Design review of the part built by this model. Coordinates are the model's own, in mm. A direction names the side the tool comes from. Coordinates: 2 decimals unless noted, no trailing zeros. Order: outer loops, then holes, each group sorted by start corner. A loop starts at its lowest first (then second) coordinate and runs counter-clockwise, first axis right, second up. Notation, with made-up numbers: M -32.5,54.25 L 17.5,54.25 A36 ccw 17.5,91.25 Z; hole C -14,67.25 d10. An arc over 180 degrees is marked long. Answer in a Markdown table with one row per item.
from build123d import *

# Parameters (mm, degrees)
PAD_DEPTH           = 50
PAD001_DEPTH        = 50
CHAMFER_SIZE        = 5
SKETCH002_R         = 6
POCKET_DEPTH        = 30
SKETCH015_R         = 6
POCKET005_DEPTH     = 292.6279206635
LINEARPATTERN_COUNT = 4
LINEARPATTERN_PITCH = 166.6666666667


with BuildPart() as part:
    # Sketch → Pad (new body)
    with BuildSketch(Plane.XY):
        with BuildLine():
            Line((-447.460817474, 354.8217734667), (19.5015988359, 27.8511695058))
            ThreePointArc((34, 0), (30.1583683281, 15.69945285), (19.5015988359, 27.8511695058))
            Line((28, 0), (34, 0))
            ThreePointArc((28, 0), (24.836303329, 12.9289611706), (16.0601402178, 22.9362572401))
            Line((16.0601402178, 22.9362572401), (-450.9022760922, 349.906861201))
            Line((-450.9022760922, 349.906861201), (-447.460817474, 354.8217734667))
        make_face()
    extrude(amount=PAD_DEPTH)

    # Sketch001 → Pad001 (join)
    with BuildSketch(Plane.XY):
        Polygon((-94.6057566753, 107.75), (-103.1746447158, 113.75), (-1.7405688034, 113.75), (-1.7405688034, 107.75), align=None)
        Polygon((-113.171680763, 120.75), (-121.7405688034, 126.75), (-1.7405688034, 126.75), (-1.7405688034, 120.75), align=None)
    extrude(amount=PAD001_DEPTH)

    # Chamfer
    chamfer_edges = [part.edges().sort_by_distance(p)[0] for p in [
        (-1.740569, 123.75, 50),
        (-1.740569, 110.75, 50),
        (-1.740569, 110.75, 0),
        (-1.740569, 123.75, 0),
    ]]
    chamfer(chamfer_edges, length=CHAMFER_SIZE)

    # Sketch002 (on Face1 of Chamfer) → Pocket (cut)
    with BuildSketch(Plane(origin=(0, 126.75, 0), x_dir=(-1, 0, 0), z_dir=(0, 1, 0))):
        with Locations((26.7405688034, 25.24131)):
            Circle(SKETCH002_R)
    extrude(amount=-POCKET_DEPTH, mode=Mode.SUBTRACT)

    # Sketch015 → Pocket005 (cut, through all)
    with BuildSketch(Plane(origin=(19.5015988359, 27.8511695058, 0), x_dir=(-0.8191520443, 0.5735764364, 0), z_dir=(0.5735764364, 0.8191520443, 0))):
        with Locations((550.0558517379, 25)):
            Circle(SKETCH015_R)
    pocket005 = extrude(amount=-POCKET005_DEPTH, mode=Mode.SUBTRACT)

    # LinearPattern: Pocket005 ×4
    with Locations(*[Vector(0.8191520443, -0.5735764364, 0) * (i * LINEARPATTERN_PITCH) for i in range(1, LINEARPATTERN_COUNT)]):
        add(pocket005, mode=Mode.SUBTRACT)


solid = part.part
(1) Insertion check: pin 1 Ø5 at (y, z) = (149, 43.5) entering from -X; pin 2 Ø6 at (x, z) = (-308, 32.5) entering from +Y; pin 3 Ø11 at (x, z) = (-26.74, 25.24) entering from +Y. Each pin has a flat end and moves straight along its axis. Give the tip position at first contact, or say it passes through.
Return value:
| item | result |
|---|---|
| pin 1 | stops at x = -167.55 |
| pin 2 | stops at y = 259.27 |
| pin 3 | stops at y = 64.08 |
(2) Add section A-A, the plane y = 83. Give the boundary of the cut face in (x, z), and give its area (3 significant figures).
Return value:
| item | result |
|---|---|
| outline | M -69.72,0 L -59.26,0 L -59.26,50 L -69.72,50 Z |
| area | 523 mm2 |
(3) Add section B-B, the plane x = -413. Give the boundary of the cut face in (y, z).
Return value:
| item | result |
|---|---|
| outline | M 323.37,0 L 330.69,0 L 330.69,50 L 323.37,50 Z |
(4) For line 1 along Y through (x, z) = (-55, 34.5); line 2 along Y through (x, z) = (-67, 28.5); line 3 along X through (y, z) = (72, 14), list the stretches that pass through material, from the lowest coordinate up. Write a range as from..to.
Return value:
| item | result |
|---|---|
| line 1 | y = 72.69..80.02, 107.75..113.75, 120.75..126.75 |
| line 2 | y = 81.1..88.42, 107.75..113.75, 120.75..126.75 |
| line 3 | x = -54.01..-43.55 |
(5) For faces 4 (the cylindrical face through (-22.32, 110.79, 29.3)), 5 (the flat face through (-63, 126.75, 25)), 6 (the flat face through (-53, 113.75, 25)), list the 3-axis set-ups (+Z, -Z, +X, -X, +Y, -Y) from which the entire face can be reached by the end or side of a thin tool; tool diameter is ignored.
Return value:
| item | result |
|---|---|
| face 4 | +Y |
| face 5 | +Z, -Z, +X, +Y |
| face 6 | +Z, -Z, +X |
(6) Draft analysis for pull direction Y (two halves, no side actions). For faces 1 (the flat face through (-286.88, 242.38, 24.65)), 2 (the cylindrical face through (24.923, 12.762, 24.65)), 3 (the flat face through (-108.243, 117.299, 24.65)), state which applies: pulls with the +Y half, pulls with the -Y half, needs draft (parallel to the pull), parting line crosses it, or undercut.
Return value:
| item | result |
|---|---|
| face 1 | pulls with the +Y half |
| face 2 | pulls with the -Y half |
| face 3 | undercut |
